Check sheet for the modelled part. Datum: model origin and axes. Units: mm. A direction names the side the tool comes from. Round coordinates to 2 decimals unless told otherwise and drop trailing zeros. One line per item, written item: value.
from build123d import *

# Parameters (mm, degrees)
SKETCH1_W           = 127.76
SKETCH1_H           = 85.48
BOSS_EXTRUDE1_DEPTH = 14
SKETCH6_R           = 3.5
CUT_EXTRUDE1_DEPTH  = 8


with BuildPart() as part:
    # Sketch1 → Boss-Extrude1 (new body)
    with BuildSketch(Plane(origin=(0, 0, 0), x_dir=(1, 0, 0), z_dir=(0, 1, 0))):
        with Locations((63.88, 42.74)):
            Rectangle(SKETCH1_W, SKETCH1_H)
    extrude(amount=BOSS_EXTRUDE1_DEPTH)

    # Sketch6 → Cut-Extrude1 (cut)
    with BuildSketch(Plane(origin=(0, 14, 0), x_dir=(1, 0, 0), z_dir=(0, 1, 0))):
        with Locations(Location((59.38, 47.24, 0), (0, 0, 270))):
            Circle(SKETCH6_R)
        with Locations(Location((14.38, 38.24, 0), (0, 0, 90))):
            Circle(SKETCH6_R)
        with Locations(Location((23.38, 38.24, 0), (0, 0, 90))):
            Circle(SKETCH6_R)
        with Locations(Location((32.38, 38.24, 0), (0, 0, 90))):
            Circle(SKETCH6_R)
        with Locations(Location((50.38, 47.24, 0), (0, 0, 270))):
            Circle(SKETCH6_R)
        with Locations(Location((41.38, 47.24, 0), (0, 0, 270))):
            Circle(SKETCH6_R)
        with Locations(Location((32.38, 47.24, 0), (0, 0, 270))):
            Circle(SKETCH6_R)
        with Locations(Location((23.38, 47.24, 0), (0, 0, 270))):
            Circle(SKETCH6_R)
        with Locations(Location((14.38, 47.24, 0), (0, 0, 270))):
            Circle(SKETCH6_R)
        with Locations(Location((41.38, 38.24, 0), (0, 0, 90))):
            Circle(SKETCH6_R)
        with Locations(Location((50.38, 38.24, 0), (0, 0, 90))):
            Circle(SKETCH6_R)
        with Locations(Location((59.38, 38.24, 0), (0, 0, 90))):
            Circle(SKETCH6_R)
        with Locations(Location((68.38, 38.24, 0), (0, 0, 270))):
            Circle(SKETCH6_R)
        with Locations(Location((77.38, 38.24, 0), (0, 0, 270))):
            Circle(SKETCH6_R)
        with Locations(Location((86.38, 38.24, 0), (0, 0, 270))):
            Circle(SKETCH6_R)
        with Locations(Location((113.38, 47.24, 0), (0, 0, 90))):
            Circle(SKETCH6_R)
        with Locations(Location((104.38, 47.24, 0), (0, 0, 90))):
            Circle(SKETCH6_R)
        with Locations(Location((95.38, 47.24, 0), (0, 0, 90))):
            Circle(SKETCH6_R)
        with Locations(Location((86.38, 47.24, 0), (0, 0, 90))):
            Circle(SKETCH6_R)
        with Locations(Location((77.38, 47.24, 0), (0, 0, 90))):
            Circle(SKETCH6_R)
        with Locations(Location((95.38, 38.24, 0), (0, 0, 270))):
            Circle(SKETCH6_R)
        with Locations(Location((104.38, 38.24, 0), (0, 0, 270))):
            Circle(SKETCH6_R)
        with Locations(Location((113.38, 38.24, 0), (0, 0, 270))):
            Circle(SKETCH6_R)
        with Locations(Location((68.38, 47.24, 0), (0, 0, 90))):
            Circle(SKETCH6_R)
        with Locations(Location((59.38, 56.24, 0), (0, 0, 270))):
            Circle(SKETCH6_R)
        with Locations(Location((50.38, 56.24, 0), (0, 0, 270))):
            Circle(SKETCH6_R)
        with Locations(Location((41.38, 56.24, 0), (0, 0, 270))):
            Circle(SKETCH6_R)
        with Locations(Location((32.38, 56.24, 0), (0, 0, 270))):
            Circle(SKETCH6_R)
        with Locations(Location((23.38, 56.24, 0), (0, 0, 270))):
            Circle(SKETCH6_R)
        with Locations(Location((14.38, 56.24, 0), (0, 0, 270))):
            Circle(SKETCH6_R)
        with Locations(Location((113.38, 56.24, 0), (0, 0, 90))):
            Circle(SKETCH6_R)
        with Locations(Location((104.38, 56.24, 0), (0, 0, 90))):
            Circle(SKETCH6_R)
        with Locations(Location((95.38, 56.24, 0), (0, 0, 90))):
            Circle(SKETCH6_R)
        with Locations(Location((86.38, 56.24, 0), (0, 0, 90))):
            Circle(SKETCH6_R)
        with Locations(Location((77.38, 56.24, 0), (0, 0, 90))):
            Circle(SKETCH6_R)
        with Locations(Location((68.38, 56.24, 0), (0, 0, 90))):
            Circle(SKETCH6_R)
        with Locations(Location((59.38, 65.24, 0), (0, 0, 270))):
            Circle(SKETCH6_R)
        with Locations(Location((50.38, 65.24, 0), (0, 0, 270))):
            Circle(SKETCH6_R)
        with Locations(Location((41.38, 65.24, 0), (0, 0, 270))):
            Circle(SKETCH6_R)
        with Locations(Location((32.38, 65.24, 0), (0, 0, 270))):
            Circle(SKETCH6_R)
        with Locations(Location((23.38, 65.24, 0), (0, 0, 270))):
            Circle(SKETCH6_R)
        with Locations(Location((14.38, 65.24, 0), (0, 0, 270))):
            Circle(SKETCH6_R)
        with Locations(Location((113.38, 65.24, 0), (0, 0, 90))):
            Circle(SKETCH6_R)
        with Locations(Location((104.38, 65.24, 0), (0, 0, 90))):
            Circle(SKETCH6_R)
        with Locations(Location((95.38, 65.24, 0), (0, 0, 90))):
            Circle(SKETCH6_R)
        with Locations(Location((86.38, 65.24, 0), (0, 0, 90))):
            Circle(SKETCH6_R)
        with Locations(Location((77.38, 65.24, 0), (0, 0, 90))):
            Circle(SKETCH6_R)
        with Locations(Location((68.38, 65.24, 0), (0, 0, 90))):
            Circle(SKETCH6_R)
        with Locations(Location((59.38, 74.24, 0), (0, 0, 270))):
            Circle(SKETCH6_R)
        with Locations(Location((50.38, 74.24, 0), (0, 0, 270))):
            Circle(SKETCH6_R)
        with Locations(Location((41.38, 74.24, 0), (0, 0, 270))):
            Circle(SKETCH6_R)
        with Locations(Location((32.38, 74.24, 0), (0, 0, 270))):
            Circle(SKETCH6_R)
        with Locations(Location((23.38, 74.24, 0), (0, 0, 270))):
            Circle(SKETCH6_R)
        with Locations(Location((14.38, 74.24, 0), (0, 0, 270))):
            Circle(SKETCH6_R)
        with Locations(Location((113.38, 74.24, 0), (0, 0, 90))):
            Circle(SKETCH6_R)
        with Locations(Location((104.38, 74.24, 0), (0, 0, 90))):
            Circle(SKETCH6_R)
        with Locations(Location((95.38, 74.24, 0), (0, 0, 90))):
            Circle(SKETCH6_R)
        with Locations(Location((86.38, 74.24, 0), (0, 0, 90))):
            Circle(SKETCH6_R)
        with Locations(Location((77.38, 74.24, 0), (0, 0, 90))):
            Circle(SKETCH6_R)
        with Locations(Location((68.38, 74.24, 0), (0, 0, 90))):
            Circle(SKETCH6_R)
        with Locations(Location((14.38, 29.24, 0), (0, 0, 90))):
            Circle(SKETCH6_R)
        with Locations(Location((23.38, 29.24, 0), (0, 0, 90))):
            Circle(SKETCH6_R)
        with Locations(Location((32.38, 29.24, 0), (0, 0, 90))):
            Circle(SKETCH6_R)
        with Locations(Location((41.38, 29.24, 0), (0, 0, 90))):
            Circle(SKETCH6_R)
        with Locations(Location((50.38, 29.24, 0), (0, 0, 90))):
            Circle(SKETCH6_R)
        with Locations(Location((59.38, 29.24, 0), (0, 0, 90))):
            Circle(SKETCH6_R)
        with Locations(Location((68.38, 29.24, 0), (0, 0, 270))):
            Circle(SKETCH6_R)
        with Locations(Location((77.38, 29.24, 0), (0, 0, 270))):
            Circle(SKETCH6_R)
        with Locations(Location((86.38, 29.24, 0), (0, 0, 270))):
            Circle(SKETCH6_R)
        with Locations(Location((95.38, 29.24, 0), (0, 0, 270))):
            Circle(SKETCH6_R)
        with Locations(Location((104.38, 29.24, 0), (0, 0, 270))):
            Circle(SKETCH6_R)
        with Locations(Location((113.38, 29.24, 0), (0, 0, 270))):
            Circle(SKETCH6_R)
        with Locations(Location((14.38, 20.24, 0), (0, 0, 90))):
            Circle(SKETCH6_R)
        with Locations(Location((23.38, 20.24, 0), (0, 0, 90))):
            Circle(SKETCH6_R)
        with Locations(Location((32.38, 20.24, 0), (0, 0, 90))):
            Circle(SKETCH6_R)
        with Locations(Location((41.38, 20.24, 0), (0, 0, 90))):
            Circle(SKETCH6_R)
        with Locations(Location((50.38, 20.24, 0), (0, 0, 90))):
            Circle(SKETCH6_R)
        with Locations(Location((59.38, 20.24, 0), (0, 0, 90))):
            Circle(SKETCH6_R)
        with Locations(Location((68.38, 20.24, 0), (0, 0, 270))):
            Circle(SKETCH6_R)
        with Locations(Location((77.38, 20.24, 0), (0, 0, 270))):
            Circle(SKETCH6_R)
        with Locations(Location((86.38, 20.24, 0), (0, 0, 270))):
            Circle(SKETCH6_R)
        with Locations(Location((95.38, 20.24, 0), (0, 0, 270))):
            Circle(SKETCH6_R)
        with Locations(Location((104.38, 20.24, 0), (0, 0, 270))):
            Circle(SKETCH6_R)
        with Locations(Location((113.38, 20.24, 0), (0, 0, 270))):
            Circle(SKETCH6_R)
        with Locations(Location((14.38, 11.24, 0), (0, 0, 90))):
            Circle(SKETCH6_R)
        with Locations(Location((23.38, 11.24, 0), (0, 0, 90))):
            Circle(SKETCH6_R)
        with Locations(Location((32.38, 11.24, 0), (0, 0, 90))):
            Circle(SKETCH6_R)
        with Locations(Location((41.38, 11.24, 0), (0, 0, 90))):
            Circle(SKETCH6_R)
        with Locations(Location((50.38, 11.24, 0), (0, 0, 90))):
            Circle(SKETCH6_R)
        with Locations(Location((59.38, 11.24, 0), (0, 0, 90))):
            Circle(SKETCH6_R)
        with Locations(Location((68.38, 11.24, 0), (0, 0, 270))):
            Circle(SKETCH6_R)
        with Locations(Location((77.38, 11.24, 0), (0, 0, 270))):
            Circle(SKETCH6_R)
        with Locations(Location((86.38, 11.24, 0), (0, 0, 270))):
            Circle(SKETCH6_R)
        with Locations(Location((95.38, 11.24, 0), (0, 0, 270))):
            Circle(SKETCH6_R)
        with Locations(Location((104.38, 11.24, 0), (0, 0, 270))):
            Circle(SKETCH6_R)
        with Locations(Location((113.38, 11.24, 0), (0, 0, 270))):
            Circle(SKETCH6_R)
    extrude(amount=-CUT_EXTRUDE1_DEPTH, mode=Mode.SUBTRACT)


solid = part.part
Item 1: Tool access check on faces 1 (the flat face through (63, 14, -43)), 2 (the flat face through (104, 6, -47)). Record the directions out of +Z, -Z, +X, -X, +Y, -Y that give a thin tool (end or side, any length) a straight path to the whole face; none if there is none.
Result set:
face 1: +Z, -Z, +X, -X, +Y
face 2: +Y
Item 2: Sectioned sample at A-A (y = 11.25). State how many separate pieces and enclosed holes the cut face has, then the cut area to 3 significant figures.
Result set:
separate pieces: 1
enclosed holes: 96
area: 7,230 mm^2
Item 3: Material ranges on line 1 along Y through (x, z) = (78, -77), recorded low to high.
Result set:
line 1: 0 to 6
Item 4: Depth check by flat-ended pin: pin 1 (8 mm diameter, centred on x = 32.38, z = -20.24, fed in from +Y); pin 2 (2 mm diameter, centred on x = 78.5, z = -31, fed in from +Y). Enter the tip coordinate at first touch or a pass-through.
Result set:
pin 1: y = 14
pin 2: y = 6
